Geometry: final body of the model. Coordinates: model frame, mm. Face numbers are marked on the shaded views. A direction names the side the tool comes from. Round coordinates to 2 decimals unless told otherwise and drop trailing zeros. Write each loop counter-clockwise with the first axis right and the second up, starting at its lowest first coordinate (ties: lowest second). Pieces come first, ordered by that corner, then holes. Notation, with made-up numbers: (-28.75, 40.5) -> (1.25, 40.5) arc R9 ccw to (1.25, 45.5) -> close; hole circle Ø6 at (64, 43.5). An arc over 180 degrees is marked (long way). Use one line per item in the form item = value. Start each with the question number.
1. Draft query along X for the marked faces 3, 4 and 5. Return one class per face: pulls with the +X half, pulls with the -X half, needs draft (parallel to the pull), parting line crosses it, or undercut.
2. Pin query (flat end, axial travel): pin 1 Ø1 at (x, z) = (0, 0.5) entering from -Y. Return the tip coordinate at first contact, or that it passes through.
3. Line query: L1, parallel to X at y = -3.45, z = -3.25; L2, parallel to Z at x = -2, y = -4.2; L3, parallel to Z at x = -1.25, y = -1.5. Output: solid intervals per line, ascending.
4. Cut plane B-B, the plane z = 2. Return the cut outline in (x, y).
5. Reachability of the marked faces 1 and 2 from +Z, -Z, +X, -X, +Y, -Y: full face, straight path, thin tool, end or side. Return the list, or none.
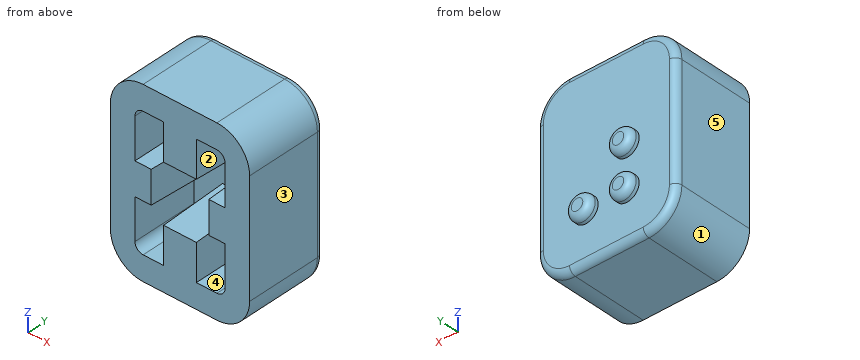
```python
from build123d import *

# Parameters (mm, degrees)
BOSS_EXTRUDE1_DEPTH = 5
SKETCH1_3_R         = 0.75
BOSS_EXTRUDE2_DEPTH = 0.6
FILLET2_R           = 0.4
SHELL1_START        = -5
SHELL1_DEPTH        = 4
BOSS_EXTRUDE4_DEPTH = 4
SKETCH4_W           = 3.1
SKETCH4_H           = 3.1
CUT_EXTRUDE1_DEPTH  = 9.019507466
CUT_EXTRUDE1_DRAFT  = -3


# Read off the part's stored shape, not the designer's step: Shell1
with BuildPart() as part:
    # Sketch1 → Boss-Extrude1 (new body)
    with BuildSketch(Plane(origin=(0, 0, 0), x_dir=(1, 0, 0), z_dir=(0, 1, 0))):
        with BuildLine():
            Line((-2.25, -5.5), (2.25, -5.5))
            ThreePointArc((2.25, -5.5), (3.664213562, -4.914213562), (4.25, -3.5))
            Line((4.25, -3.5), (4.25, 3.5))
            ThreePointArc((4.25, 3.5), (3.664213562, 4.914213562), (2.25, 5.5))
            Line((2.25, 5.5), (-2.25, 5.5))
            ThreePointArc((-2.25, 5.5), (-3.664213562, 4.914213562), (-4.25, 3.5))
            Line((-4.25, 3.5), (-4.25, -3.5))
            ThreePointArc((-4.25, -3.5), (-3.664213562, -4.914213562), (-2.25, -5.5))
        make_face()
    extrude(amount=-BOSS_EXTRUDE1_DEPTH)

    # Sketch1<3> → Boss-Extrude2 (add)
    with BuildSketch(Plane(origin=(0, 0, 0), x_dir=(1, 0, 0), z_dir=(0, 1, 0))):
        with Locations(Location((1.25, 2.5, 0), (0, 0, 270))):
            Circle(SKETCH1_3_R)
        with Locations(Location((-1.25, 0, 0), (0, 0, 270))):
            Circle(SKETCH1_3_R)
        with Locations(Location((-1.25, 2.5, 0), (0, 0, 270))):
            Circle(SKETCH1_3_R)
    extrude(amount=BOSS_EXTRUDE2_DEPTH)

    # Fillet2
    fillet2_edges = [part.edges().sort_by_distance(p)[0] for p in [
        (3.664213562, 0, -4.914213562),
        (4.25, 0, 0),
        (3.664213562, 0, 4.914213562),
        (0, 0, 5.5),
        (-1.25, 0.6, -3.25),
        (-1.25, 0.6, -0.75),
        (1.25, 0.6, -3.25),
        (-3.664213562, 0, 4.914213562),
        (-4.25, 0, 0),
        (-3.664213562, 0, -4.914213562),
        (0, 0, -5.5),
    ]]
    fillet(fillet2_edges, radius=FILLET2_R)

    # Shell1 outline → Shell1 (cut)
    with BuildSketch(Plane(origin=(0, 0, 0), x_dir=(1, 0, 0), z_dir=(0, 1, 0)).offset(SHELL1_START)):
        with BuildLine():
            ThreePointArc((-2.75, -3.5), (-2.603553391, -3.853553391), (-2.25, -4))
            Line((-2.25, -4), (2.25, -4))
            ThreePointArc((2.25, -4), (2.603553391, -3.853553391), (2.75, -3.5))
            Line((2.75, -3.5), (2.75, 3.5))
            ThreePointArc((2.75, 3.5), (2.603553391, 3.853553391), (2.25, 4))
            Line((2.25, 4), (-2.25, 4))
            ThreePointArc((-2.25, 4), (-2.603553391, 3.853553391), (-2.75, 3.5))
            Line((-2.75, 3.5), (-2.75, -3.5))
        make_face()
    extrude(amount=SHELL1_DEPTH, mode=Mode.SUBTRACT)

    # Sketch3 → Boss-Extrude4 (add)
    with BuildSketch(Plane.XZ.offset(1)):
        Polygon((-1, 4), (1, 4), (1, 1), (2.75, 1), (2.75, -1), (1, -1), (1, -4), (-1, -4), (-1, -1), (-2.75, -1), (-2.75, 1), (-1, 1), align=None)
    extrude(amount=BOSS_EXTRUDE4_DEPTH)


with BuildPart() as cut_extrude1_tool:
    # Sketch4 → Cut-Extrude1 (with draft: the straight prism first)
    with BuildSketch(Plane.XZ.offset(1)):
        Rectangle(SKETCH4_W, SKETCH4_H)
    extrude(amount=CUT_EXTRUDE1_DEPTH)
    # Cut-Extrude1: the draft: its side faces are tilted about the plane it starts from
    cut_extrude1_sides = [cut_extrude1_tool.faces().sort_by_distance(p)[0] for p in [
        (0, -5.509753733, -1.55),
        (1.55, -5.509753733, 0),
        (0, -5.509753733, 1.55),
        (-1.55, -5.509753733, 0),
    ]]
    draft(cut_extrude1_sides, Plane.XZ.offset(1), CUT_EXTRUDE1_DRAFT)


with BuildPart() as part_1:
    add(part.part)

    # Cut-Extrude1: cut by cut_extrude1_tool
    add(cut_extrude1_tool.part, mode=Mode.SUBTRACT)


solid = part_1.part
```
Outcome:
q1.face_3 = pulls with the +X half
q1.face_4 = undercut
q1.face_5 = pulls with the -X half
q2.pin_1 = -1
q3.L1 = -4.25 to -2.75, -1 to 1, 2.75 to 4.25
q3.L2 = -5.5 to -4, -1 to 1, 4 to 5.5
q3.L3 = -5.5 to -4, 4 to 5.5
q4.outline = (-4.25, -5) -> (-2.75, -5) -> (-2.75, -1) -> (-1, -1) -> (-1, -5) -> (1, -5) -> (1, -1) -> (2.75, -1) -> (2.75, -5) -> (4.25, -5) -> (4.25, -0.4) arc R0.4 ccw to (3.85, 0) -> (-3.85, 0) arc R0.4 ccw to (-4.25, -0.4) -> close
q5.face_1 = -Z, -X, +Y, -Y
q5.face_2 = -Y
